```python
from build123d import *

# Parameters (mm, degrees)
BOSS_EXTRUDE1_DEPTH = 25.4
SKETCH2_R           = 3.175
CUT_EXTRUDE1_DEPTH  = 4.175
SKETCH3_R           = 3.175
CUT_EXTRUDE2_DEPTH  = 4.175


with BuildPart() as part:
    # Sketch1 → Boss-Extrude1 (new body)
    with BuildSketch(Plane.XY):
        Polygon((0, 0), (0, 38.1), (3.175, 38.1), (3.175, 3.175), (38.1, 3.175), (38.1, 0), align=None)
    extrude(amount=BOSS_EXTRUDE1_DEPTH)

    # Sketch2 → Cut-Extrude1 (cut, through all)
    with BuildSketch(Plane(origin=(0, 3.175, 0), x_dir=(1, 0, 0), z_dir=(0, 1, 0))):
        with Locations((19.05, -12.7)):
            Circle(SKETCH2_R)
    extrude(amount=-CUT_EXTRUDE1_DEPTH, mode=Mode.SUBTRACT)

    # Sketch3 → Cut-Extrude2 (cut, through all)
    with BuildSketch(Plane(origin=(3.175, 0, 0), x_dir=(0, 0, -1), z_dir=(1, 0, 0))):
        with Locations((-12.7, 28.575)):
            Circle(SKETCH3_R)
    extrude(amount=-CUT_EXTRUDE2_DEPTH, mode=Mode.SUBTRACT)


solid = part.part
```
Geometry check sheet. Reference: the model listing, model coordinates, mm. A direction names the side the tool comes from. Coordinates: 2 decimals unless noted, no trailing zeros. Loops run counter-clockwise (first coordinate to the right, second up) from the corner with the lowest first, then second, coordinate; pieces in that order, holes last. Notation, with made-up numbers: (84, 69.5) - (103, 69.5) arc R17 ccw to (103, 76.5) - close; hole circle Ø10 at (-32, -22.75). An arc over 180 degrees is marked (long way). One line per item, written item: value. Start each with the question number.
(1) Cross-section at B-B on z = 12.7. Enter the section's corners in (x, y) (3 decimals), plus the area to 3 significant figures.
(2) Cross-section at A-A on x = 19.05. Enter the section's corners in (y, z) (3 decimals).
(3) Material ranges on line 1 (Y direction, x = 1.75, z = 12.7); line 2 (Z direction, x = 19.05, y = 2.4) (3 decimals); line 3 (Y direction, x = 26, z = 3.75) (3 decimals), recorded low to high. Write a range as [from, to].
(4) Cross-section at C-C on y = 29.5. Enter the section's corners in (x, z) (3 decimals), plus the area to 3 significant figures.
(5) Depth check by flat-ended pin: P1, Ø5, axis at x = 8, z = 21, coming from the +Y side (3 decimals); P2, Ø5, axis at y = 28.575, z = 12.7, coming from the +X side; P3, Ø12.5, axis at y = 12, z = 16.5, coming from the +X side (3 decimals). Enter the tip coordinate at first touch or a pass-through.
(6) Tool access check on faces 4 (the cylindrical face through (16.53, 1.61, 14.63)), 5 (the flat face through (24, 3.175, 13)). Record the directions out of +Z, -Z, +X, -X, +Y, -Y that give a thin tool (end or side, any length) a straight path to the whole face; none if there is none.
(7) Cross-section at D-D on y = 9. Enter the section's corners in (x, z) (3 decimals).
(8) Mould release check, pull along Z, two halves, no side actions. Record for faces 1 (the flat face through (11, 2, 25.4)), 2 (the flat face through (38.1, 2, 13)), 3 (the cylindrical face through (1.61, 25.476, 13.388)): released by +Z, released by -Z, zero draft, split by the parting line, or undercut.
Results below:
1. outline: (0, 0) - (15.875, 0) - (15.875, 3.175) - (3.175, 3.175) - (3.175, 25.4) - (0, 25.4) - close; (0, 31.75) - (3.175, 31.75) - (3.175, 38.1) - (0, 38.1) - close; (22.225, 0) - (38.1, 0) - (38.1, 3.175) - (22.225, 3.175) - close
1. area: 192 mm2
2. outline: (0, 0) - (3.175, 0) - (3.175, 9.525) - (0, 9.525) - close; (0, 15.875) - (3.175, 15.875) - (3.175, 25.4) - (0, 25.4) - close
3. line 1: y = [0, 25.4], [31.75, 38.1]
3. line 2: z = [0, 9.525], [15.875, 25.4]
3. line 3: y = [0, 3.175]
4. outline: (0, 0) - (3.175, 0) - (3.175, 9.663) - (0, 9.663) - close; (0, 15.737) - (3.175, 15.737) - (3.175, 25.4) - (0, 25.4) - close
4. area: 61.4 mm2
5. P1: stops at y = 3.175
5. P2: passes through
5. P3: stops at x = 3.175
6. face 4: +Y, -Y
6. face 5: +Z, -Z, +X, +Y
7. outline: (0, 0) - (3.175, 0) - (3.175, 25.4) - (0, 25.4) - close
8. face 1: released by +Z
8. face 2: zero draft
8. face 3: undercut
